from build123d import *

# Parameters (mm, degrees)
SKETCH037_W     = 80
SKETCH037_H     = 87
PAD015_DEPTH    = 3
SKETCH038_R     = 1.6
SKETCH038_R_2   = 5
POCKET021_DEPTH = 3.001
CHAMFER019_SIZE = 2
SKETCH044_R     = 1.6
POCKET025_DEPTH = 3.001
POCKET030_DEPTH = 3.001
CHAMFER029_SIZE = 1


with BuildPart() as part:
    # Sketch037 → Pad015 (new body)
    with BuildSketch(Plane.XZ):
        with Locations((0, 7.5)):
            Rectangle(SKETCH037_W, SKETCH037_H)
    extrude(amount=-PAD015_DEPTH)

    # Sketch038 → Pocket021 (cut, through all)
    with BuildSketch(Plane.XZ):
        with Locations((-12.5, 40)):
            Circle(SKETCH038_R)
        with Locations((12.5, 40)):
            Circle(SKETCH038_R)
        with Locations((-24, 40)):
            Circle(SKETCH038_R_2)
        with Locations((24, 40)):
            Circle(SKETCH038_R_2)
    extrude(amount=-POCKET021_DEPTH, mode=Mode.SUBTRACT)

    # Chamfer019
    chamfer019_edges = [part.edges().sort_by_distance(p)[0] for p in [
        (40, 1.5, 51),
        (-40, 1.5, 51),
        (40, 1.5, -36),
        (-40, 1.5, -36),
    ]]
    chamfer(chamfer019_edges, length=CHAMFER019_SIZE)

    # Sketch044 → Pocket025 (cut, through all)
    with BuildSketch(Plane.XZ):
        with Locations((24, -31)):
            Circle(SKETCH044_R)
        with Locations((-24, -31)):
            Circle(SKETCH044_R)
    extrude(amount=-POCKET025_DEPTH, mode=Mode.SUBTRACT)

    # Sketch054 (on Face2 of Pocket025) → Pocket030 (cut, through all)
    with BuildSketch(Plane.XZ):
        with BuildLine():
            Line((40, 28.485281), (15.757359, 4.242641))
            ThreePointArc((15.757359, 4.242641), (15.757359, -4.242641), (24.242641, -4.242641))
            Line((40, 11.514719), (24.242641, -4.242641))
            Line((40, 28.485281), (40, 11.514719))
        make_face()
    extrude(amount=-POCKET030_DEPTH, mode=Mode.SUBTRACT)

    # Chamfer029
    chamfer029_edges = [part.edges().sort_by_distance(p)[0] for p in [
        (40, 1.5, 28.485281),
        (40, 1.5, 11.514719),
    ]]
    chamfer(chamfer029_edges, length=CHAMFER029_SIZE)


solid = part.part
Design review of the part built by this model. Coordinates are the model's own, in mm. A direction names the side the tool comes from. Round coordinates to 2 decimals unless told otherwise and drop trailing zeros. Loops run counter-clockwise (first coordinate to the right, second up) from the corner with the lowest first, then second, coordinate; pieces in that order, holes last. Notation, with made-up numbers: M 59,35.25 L 95,35.25 A7 cw 95,46.25 Z; hole C -30.75,83 d11. An arc over 180 degrees is marked long. Answer as a JSON object with one key per item and string values.
Item 1: Wall thickness on L1, parallel to Z at x = -24, y = 0.95; L2, parallel to Z at x = 24, y = 2.35; L3, parallel to Z at x = 12.5, y = 1.65: over which ranges is each line inside the solid? List them lowest first. Write a range as from..to.
Answer sheet:
{"L1": "z = -36..-32.6, -29.4..35, 45..51", "L2": "z = -36..-32.6, -29.4..-4.47, 12.49..35, 45..51", "L3": "z = -36..38.4, 41.6..51"}
Item 2: The part is to be moulded in two halves that separate along Z. For faces 1 (the flat face through (-40, 1, 7)), 2 (the cylindrical face through (-23.26, 1.48, -32.42)), 3 (the flat face through (39, 1, 50)), say which applies: pulls with the +Z half, pulls with the -Z half, needs draft (parallel to the pull), parting line crosses it, or undercut.
Answer sheet:
{"face 1": "needs draft", "face 2": "undercut", "face 3": "pulls with the +Z half"}
Item 3: Machinability: for faces 4 (the flat face through (31.873, 1.479, 3.388)), 5 (the flat face through (-1, 0, 8)), which of the approach directions +Z, -Z, +X, -X, +Y, -Y give a long, thin tool a straight path to every point of the face, cutting with its end or side? Answer none if there is none.
Answer sheet:
{"face 4": "+Y, -Y", "face 5": "+Z, -Z, +X, -X, -Y"}
Item 4: We need section A-A on z = -31. Give the boundary of the cut face in (x, y), and give its area (3 significant figures).
Answer sheet:
{"outline": "M -40,0 L -25.6,0 L -25.6,3 L -40,3 Z; M -22.4,0 L 22.4,0 L 22.4,3 L -22.4,3 Z; M 25.6,0 L 40,0 L 40,3 L 25.6,3 Z", "area": "221 mm^2"}
Item 5: We need section C-C on y = 0.9. Give the boundary of the cut face in (x, z).
Answer sheet:
{"outline": "M -40,-34 L -38,-36 L 38,-36 L 40,-34 L 40,10.51 L 39.29,10.81 L 24.24,-4.24 A6 cw 15.76,4.24 L 39.29,27.78 L 40,29.49 L 40,49 L 38,51 L -38,51 L -40,49 Z; hole C -24,40 d10; hole C -24,-31 d3.2; hole C -12.5,40 d3.2; hole C 12.5,40 d3.2; hole C 24,40 d10; hole C 24,-31 d3.2"}
Item 6: Clearance check with a flat-ended pin moving along its axis: P1, Ø9, axis at x = 24, z = 40, coming from the -Y side. State where the tip first meets the part, or that it passes through.
Answer sheet:
{"P1": "passes through"}
Item 7: We need section D-D on z = 40. Give the boundary of the cut face in (x, y), and give its area (3 significant figures).
Answer sheet:
{"outline": "M -40,0 L -29,0 L -29,3 L -40,3 Z; M -19,0 L -14.1,0 L -14.1,3 L -19,3 Z; M -10.9,0 L 10.9,0 L 10.9,3 L -10.9,3 Z; M 14.1,0 L 19,0 L 19,3 L 14.1,3 Z; M 29,0 L 40,0 L 40,3 L 29,3 Z", "area": "161 mm^2"}
Item 8: We need section B-B on x = -24. Give the boundary of the cut face in (y, z), and give its area (3 significant figures).
Answer sheet:
{"outline": "M 0,-36 L 3,-36 L 3,-32.6 L 0,-32.6 Z; M 0,-29.4 L 3,-29.4 L 3,35 L 0,35 Z; M 0,45 L 3,45 L 3,51 L 0,51 Z", "area": "221 mm^2"}
